Design review of the part built by this model. Coordinates are the model's own, in mm. Round coordinates to 2 decimals unless told otherwise and drop trailing zeros. Order: outer loops, then holes, each group sorted by start corner. A loop starts at its lowest first (then second) coordinate and runs counter-clockwise, first axis right, second up. Notation, with made-up numbers: M 81,44 L 140,44 A6 ccw 140,53 Z; hole C 79,-24 d1. An arc over 180 degrees is marked long. Write each question's results on one line, items separated by ' | '. Start each with the question number.
Item 1: Take a section at B-B, the plane z = -85. Write out the cut boundary in (x, y).
Item 2: Wall thickness on line 1 (X direction, y = 7, z = 84.5); line 2 (Z direction, x = 188, y = 1): over which ranges is each line inside the solid? List them lowest first. Write a range as [from, to].
Item 3: Clearance check with flat-ended pins moving along their axes: pin 1 (3 mm diameter, centred on x = 121.21, z = 21.21, fed in from +Y) (3 decimals); pin 2 (14.5 mm diameter, centred on x = 15, z = 85, fed in from -Y). State where each tip first meets the part, or that it passes through.
Item 4: Take a section at A-A, the plane x = 185. Write out the cut boundary in (y, z).
```python
from build123d import *

# Parameters (mm, degrees)
SKETCH1_W             = 200
SKETCH1_H             = 200
BOSS_EXTRUDE1_DEPTH   = 10
M8_CLEARANCE_HOLE1_D  = 9
M4X0_7_TAPPED_HOLE1_D = 3.3
CHAMFER1_SIZE         = 3


with BuildPart() as part:
    # Sketch1 → Boss-Extrude1 (new body)
    with BuildSketch(Plane(origin=(0, 0, 0), x_dir=(1, 0, 0), z_dir=(0, 1, 0))):
        with Locations((100, 0)):
            Rectangle(SKETCH1_W, SKETCH1_H)
    extrude(amount=BOSS_EXTRUDE1_DEPTH)

    # M8 Clearance Hole1 (through all)
    with Locations(Plane(origin=(0, 10, 0), x_dir=(-1, 0, 0), z_dir=(0, 1, 0))):
        with Locations((-15, 85), (-15, -85), (-185, -85), (-185, 85)):
            Hole(M8_CLEARANCE_HOLE1_D / 2)

    # M4x0.7 Tapped Hole1 (through all)
    with Locations(Plane(origin=(0, 10, 0), x_dir=(-1, 0, 0), z_dir=(0, 1, 0))):
        with Locations((-78.786796564, 21.213203436), (-121.213203436, 21.213203436), (-121.213203436, -21.213203436), (-78.786796564, -21.213203436)):
            Hole(M4X0_7_TAPPED_HOLE1_D / 2)

    # Chamfer1
    chamfer1_edges = [part.edges().sort_by_distance(p)[0] for p in [
        (0, 5, -100),
        (200, 5, -100),
        (200, 5, 100),
        (0, 5, 100),
    ]]
    chamfer(chamfer1_edges, length=CHAMFER1_SIZE)


solid = part.part
```
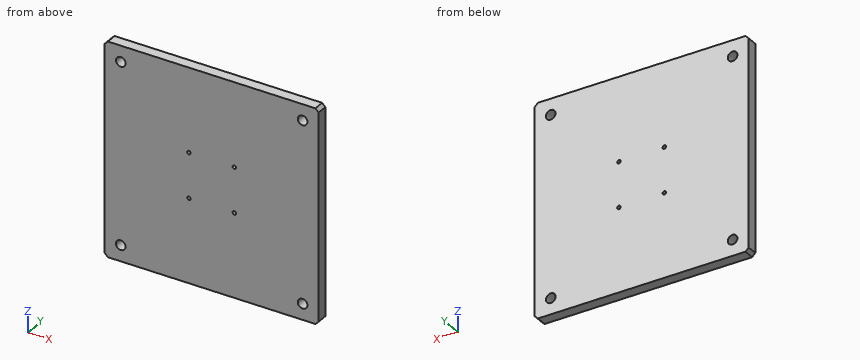
Results list:
1) outline: M 0,0 L 10.5,0 L 10.5,10 L 0,10 Z; M 19.5,0 L 180.5,0 L 180.5,10 L 19.5,10 Z; M 189.5,0 L 200,0 L 200,10 L 189.5,10 Z
2) line 1: [0, 10.53], [19.47, 180.53], [189.47, 200] | line 2: [-100, -88.35], [-81.65, 81.65], [88.35, 100]
3) pin 1: through | pin 2: y = 0
4) outline: M 0,-100 L 10,-100 L 10,-89.5 L 0,-89.5 Z; M 0,-80.5 L 10,-80.5 L 10,80.5 L 0,80.5 Z; M 0,89.5 L 10,89.5 L 10,100 L 0,100 Z
